```python
from build123d import *

# Parameters (mm, degrees)
SKIZZE1_W               = 11
SKIZZE1_H               = 10
LINEAR_AUSTRAGEN1_DEPTH = 22
SKIZZE2_R               = 2.5
LINEAR_AUSTRAGEN2_DEPTH = 8


with BuildPart() as part:
    # Skizze1 → Linear austragen1 (new body)
    with BuildSketch(Plane.XY):
        with Locations((0, 5)):
            Rectangle(SKIZZE1_W, SKIZZE1_H)
    extrude(amount=-LINEAR_AUSTRAGEN1_DEPTH)

    # Skizze2 → Linear austragen2 (add)
    with BuildSketch(Plane.XY):
        with Locations((0, 5)):
            Circle(SKIZZE2_R)
    extrude(amount=LINEAR_AUSTRAGEN2_DEPTH)


solid = part.part
```
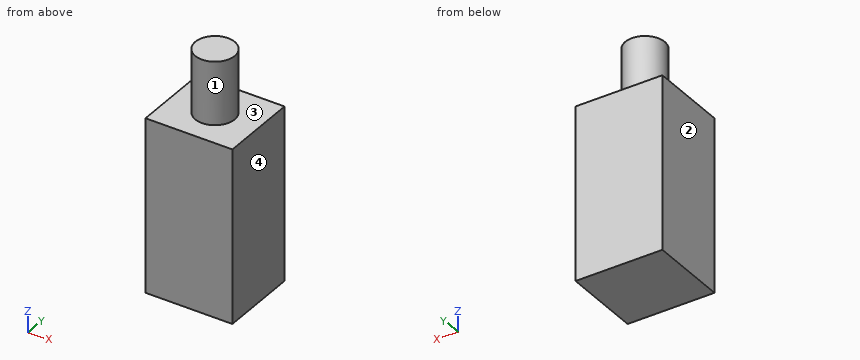
Check sheet for the modelled part. Datum: model origin and axes. Units: mm. Face numbers are marked on the shaded views. Give positions to 0.01 mm unless a question says otherwise; leave off trailing zeros. Loops run counter-clockwise (first coordinate to the right, second up) from the corner with the lowest first, then second, coordinate; pieces in that order, holes last. Notation, with made-up numbers: (25.25, -2) - (74.25, -2) arc R19 ccw to (74.25, 5) - close; hole circle Ø10 at (21.5, 26.25). An arc over 180 degrees is marked (long way). One line per question, with ' | ' between items. Start each with the question number.
1. Material ranges on line 1 along Z through (x, y) = (4.5, 9.25); line 2 along X through (y, z) = (2.75, 0.5); line 3 along X through (y, z) = (5.75, 5), recorded low to high. Write a range as [from, to].
2. Cross-section at B-B, the plane y = 5. Enter the section's corners in (x, z).
3. Cross-section at D-D, the plane y = 9. Enter the section's corners in (x, z), plus the area to 3 significant figures.
4. Gauge pin test, flat ends, axial feed: pin 1 Ø3 at (x, z) = (3, 3.5) entering from +Y; pin 2 Ø2 at (x, y) = (2, 8.5) entering from +Z. Record the tip position at first contact, or that the pin passes through.
5. Cross-section at C-C, the plane x = -3.5. Enter the section's corners in (y, z), plus the area to 3 significant figures.
6. Cross-section at A-A, the plane x = 0. Enter the section's corners in (y, z), plus the area to 3 significant figures.
7. Draft check along X on the marked faces 1, 2, 3 and 4. Enter one of: released by +X, released by -X, zero draft, split by the parting line, or undercut.
Check result:
1) line 1: z = [-22, 0] | line 2: x = [-1.09, 1.09] | line 3: x = [-2.38, 2.38]
2) outline: (-5.5, -22) - (5.5, -22) - (5.5, 0) - (2.5, 0) - (2.5, 8) - (-2.5, 8) - (-2.5, 0) - (-5.5, 0) - close
3) outline: (-5.5, -22) - (5.5, -22) - (5.5, 0) - (-5.5, 0) - close | area: 242 mm2
4) pin 1: stops at y = 7 | pin 2: stops at z = 0
5) outline: (0, -22) - (10, -22) - (10, 0) - (0, 0) - close | area: 220 mm2
6) outline: (0, -22) - (10, -22) - (10, 0) - (7.5, 0) - (7.5, 8) - (2.5, 8) - (2.5, 0) - (0, 0) - close | area: 260 mm2
7) face 1: split by the parting line | face 2: released by -X | face 3: zero draft | face 4: released by +X
